```python
from build123d import *

# Parameters (mm, degrees)
F3_DEPTH       = 7
F5_DEPTH       = 4
F5_DEPTH_BACK  = 11
F7_D           = 3.3
F7_CSINK_D     = 5
F7_CSINK_ANGLE = 90
F8_T1_DEPTH    = 38.05
F8_T3_DEPTH    = 9.5
F8_T5_DEPTH    = 12.5
F8_T7_DEPTH    = 5.25
F8_T9_DEPTH    = 5.25
F8_T11_DEPTH   = 17.5
F8_T17_DEPTH   = 39.3
F8_T21_DEPTH   = 6.5
F8_T28_DEPTH   = 39.3
F8_T32_DEPTH   = 6.5


# Not quite as in the source:
# - a fillet or chamfer that OpenCascade refuses, or shapes differently, is made with other operations: its cross-section is extruded or revolved along the edge and cut away or added


with BuildPart() as f3:
    # F2 (on Top) → F3 (new body)
    with BuildSketch(Plane.XY):
        Polygon((0, 4), (0, 0), (0.5, 0), (0.5, 1), (36.8, 1), (36.8, 0), (46.8, 0), (46.8, 4), align=None)
    extrude(amount=F3_DEPTH)

    # F4 (on face) → F5 (join, two sides)
    with BuildSketch(Plane.XY.offset(7)) as f5_sk:
        Polygon((36.8, 1), (36.8, 0), (46.8, 0), (46.8, 4), (36.8, 4), align=None)
    extrude(amount=F5_DEPTH)
    extrude(f5_sk.sketch, amount=-F5_DEPTH_BACK)

    # F7 (through all)
    with Locations(Plane(origin=(0, 4, 0), x_dir=(-1, 0, 0), z_dir=(0, 1, 0))):
        with Locations((-41.8, 8), (-41.8, -1)):
            CounterSinkHole(F7_D / 2, F7_CSINK_D / 2, counter_sink_angle=F7_CSINK_ANGLE)

    # F8: fillet of radius 0.5 on 8 edges, made by hand

    # F8_s2 → F8_t1 (cut)
    with BuildSketch(Plane.YZ.offset(-1.25)):
        with BuildLine():
            ThreePointArc((4, 6.5), (3.8535533906, 6.8535533906), (3.5, 7))
            Line((3.5, 7), (4, 7))
            Line((4, 7), (4, 6.5))
        make_face()
        with BuildLine():
            ThreePointArc((4, 0.5), (3.8535533906, 0.1464466094), (3.5, 0))
            Line((3.5, 0), (4, 0))
            Line((4, 0), (4, 0.5))
        make_face()
    extrude(amount=F8_T1_DEPTH, mode=Mode.SUBTRACT)

    # F8_s4 → F8_t3 (cut)
    with BuildSketch(Plane.XY.offset(-1.25)):
        with BuildLine():
            ThreePointArc((0, 3.5), (0.1464466094, 3.8535533906), (0.5, 4))
            Line((0.5, 4), (0, 4))
            Line((0, 4), (0, 3.5))
        make_face()
    extrude(amount=F8_T3_DEPTH, mode=Mode.SUBTRACT)

    # F8_s6 → F8_t5 (cut)
    with BuildSketch(Plane.YZ.offset(35.55)):
        with BuildLine():
            ThreePointArc((4, -3.5), (3.8535533906, -3.8535533906), (3.5, -4))
            Line((3.5, -4), (4, -4))
            Line((4, -4), (4, -3.5))
        make_face()
        with BuildLine():
            ThreePointArc((4, 10.5), (3.8535533906, 10.8535533906), (3.5, 11))
            Line((3.5, 11), (4, 11))
            Line((4, 11), (4, 10.5))
        make_face()
    extrude(amount=F8_T5_DEPTH, mode=Mode.SUBTRACT)

    # F8_s8 → F8_t7 (cut)
    with BuildSketch(Plane.XY.offset(-5.25)):
        with BuildLine():
            ThreePointArc((37.3, 4), (36.9464466094, 3.8535533906), (36.8, 3.5))
            Line((36.8, 3.5), (36.8, 4))
            Line((36.8, 4), (37.3, 4))
        make_face()
    extrude(amount=F8_T7_DEPTH, mode=Mode.SUBTRACT)

    # F8_s10 → F8_t9 (cut)
    with BuildSketch(Plane.XY.offset(7)):
        with BuildLine():
            ThreePointArc((37.3, 4), (36.9464466094, 3.8535533906), (36.8, 3.5))
            Line((36.8, 3.5), (36.8, 4))
            Line((36.8, 4), (37.3, 4))
        make_face()
    extrude(amount=F8_T9_DEPTH, mode=Mode.SUBTRACT)

    # F8_s12 → F8_t11 (cut)
    with BuildSketch(Plane.XY.offset(-5.25)):
        with BuildLine():
            ThreePointArc((46.3, 4), (46.6535533906, 3.8535533906), (46.8, 3.5))
            Line((46.8, 3.5), (46.8, 4))
            Line((46.8, 4), (46.3, 4))
        make_face()
    extrude(amount=F8_T11_DEPTH, mode=Mode.SUBTRACT)


with BuildPart() as f8_tool15:
    # F8_s16 → F8_t17 (new body)
    with BuildSketch(Plane.YZ.offset(38.05)):
        with BuildLine():
            ThreePointArc((4, 6.5), (3.8535533906, 6.8535533906), (3.5, 7))
            Line((3.5, 7), (4, 7))
            Line((4, 7), (4, 6.5))
        make_face()
    extrude(amount=-F8_T17_DEPTH)

    split(bisect_by=Plane.YZ.offset(36.8), keep=Keep.TOP)


with BuildPart() as f8_tool19:
    # F8_s20 → F8_t21 (new body)
    with BuildSketch(Plane.XY.offset(12.25)):
        with BuildLine():
            ThreePointArc((37.3, 4), (36.9464466094, 3.8535533906), (36.8, 3.5))
            Line((36.8, 3.5), (36.8, 4))
            Line((36.8, 4), (37.3, 4))
        make_face()
    extrude(amount=-F8_T21_DEPTH)

    split(bisect_by=Plane.XY.offset(7), keep=Keep.BOTTOM)


with BuildPart() as f8_tool15_1:
    add(f8_tool15.part)

    # F8_t23: intersect F8_tool19
    add(f8_tool19.part, mode=Mode.INTERSECT)


with BuildPart() as f3_1:
    add(f3.part)

    # F8_t13: cut F8_tool15
    add(f8_tool15_1.part, mode=Mode.SUBTRACT)


with BuildPart() as f8_tool26:
    # F8_s27 → F8_t28 (new body)
    with BuildSketch(Plane.YZ.offset(38.05)):
        with BuildLine():
            ThreePointArc((4, 0.5), (3.8535533906, 0.1464466094), (3.5, 0))
            Line((3.5, 0), (4, 0))
            Line((4, 0), (4, 0.5))
        make_face()
    extrude(amount=-F8_T28_DEPTH)

    split(bisect_by=Plane.YZ.offset(36.8), keep=Keep.TOP)


with BuildPart() as f8_tool30:
    # F8_s31 → F8_t32 (new body)
    with BuildSketch(Plane.XY.offset(1.25)):
        with BuildLine():
            ThreePointArc((37.3, 4), (36.9464466094, 3.8535533906), (36.8, 3.5))
            Line((36.8, 3.5), (36.8, 4))
            Line((36.8, 4), (37.3, 4))
        make_face()
    extrude(amount=-F8_T32_DEPTH)

    split(bisect_by=Plane.XY, keep=Keep.TOP)


with BuildPart() as f8_tool26_1:
    add(f8_tool26.part)

    # F8_t34: intersect F8_tool30
    add(f8_tool30.part, mode=Mode.INTERSECT)


with BuildPart() as f3_2:
    add(f3_1.part)

    # F8_t24: cut F8_tool26
    add(f8_tool26_1.part, mode=Mode.SUBTRACT)


solid = f3_2.part
```
Can you work these out from the model? Positions are in its coordinate system, mm. A direction names the side the tool comes from. Coordinates: 2 decimals unless noted, no trailing zeros. Loops run counter-clockwise (first coordinate to the right, second up) from the corner with the lowest first, then second, coordinate; pieces in that order, holes last.
Item 1: I'm going to push flat-ended pins straight in: pin 1 (1.5 mm diameter, centred on y = 2.5, z = -1.5, fed in from -X); pin 2 (1 mm diameter, centred on x = 9.5, y = 2.5, fed in from -Z); pin 3 (5.5 mm diameter, centred on x = 26, z = 4, fed in from -Y). Where does each tip first touch, or does it pass through?
Answers below:
pin 1: stops at x = 36.8
pin 2: stops at z = 0
pin 3: stops at y = 1
Item 2: Suppose I cut it at B-B (z = -1). Please give me the cut outline in (x, y).
Answers below:
outline: (36.8, 0) - (40.15, 0) - (40.15, 3.15) - (39.3, 4) - (37.3, 4) arc R0.5 ccw to (36.8, 3.5) - close; (43.45, 0) - (46.8, 0) - (46.8, 3.5) arc R0.5 ccw to (46.3, 4) - (44.3, 4) - (43.45, 3.15) - close
Item 3: Suppose I cut it at A-A (y = 0.5). Please give me the cut outline in (x, z).
Answers below:
outline: (0, 0) - (0.5, 0) - (0.5, 7) - (0, 7) - close; (36.8, -4) - (46.8, -4) - (46.8, 11) - (36.8, 11) - close; hole circle Ø3.3 at (41.8, -1); hole circle Ø3.3 at (41.8, 8)
Item 4: Suppose I cut it at C-C (z = 5). Please give me the cut outline in (x, y), then the cut area to 3 significant figures.
Answers below:
outline: (0, 0) - (0.5, 0) - (0.5, 1) - (36.8, 1) - (36.8, 0) - (46.8, 0) - (46.8, 3.5) arc R0.5 ccw to (46.3, 4) - (0.5, 4) arc R0.5 ccw to (0, 3.5) - close
area: 151 mm2
Item 5: Suppose I cut it at D-D (y = 2.4). Please give me the cut outline in (x, z), then the cut area to 3 significant figures.
Answers below:
outline: (0, 0) - (36.8, 0) - (36.8, -4) - (46.8, -4) - (46.8, 11) - (36.8, 11) - (36.8, 7) - (0, 7) - close; hole circle Ø3.3 at (41.8, -1); hole circle Ø3.3 at (41.8, 8)
area: 390 mm2
Item 6: Which directions (+Z, -Z, +X, -X, +Y, -Y) give clear straight access to the entire face, cutting with the end or side of a thin tool? Please do faces 4 (the face through (36.8, 0.6, 3.4)), 5 (the face through (18, 3, 0)), 6 (the face through (18, 1, 3)).
Answers below:
face 4: -Y
face 5: -Z, -X, +Y, -Y
face 6: +Z, -Z, -Y
Item 7: If we mould it in two halves opening along X, with no side actions, what happens to faces 1 (the face through (0.5, 0.5, 3.5)), 2 (the face through (18, 3, 7)), 3 (the face through (46.8, 2, 3))? For each: released by +X, released by -X, zero draft, split by the parting line, or undercut.
Answers below:
face 1: undercut
face 2: zero draft
face 3: released by +X
Item 8: Please list where these lines run through material, in increasing order: L1, parallel to Z at x = 41.8, y = 2.3; L2, parallel to X at y = 1.45, z = 8; L3, parallel to Z at x = 10.5, y = 3.6.
Answers below:
L1: z = -4 to -2.65, 0.65 to 6.35, 9.65 to 11
L2: x = 36.8 to 40.15, 43.45 to 46.8
L3: z = 0.01 to 6.99
